from build123d import *

# Parameters (mm, degrees)
SKETCH1_W           = 70
SKETCH1_H           = 70
SKETCH1_R           = 3.1
BOSS_EXTRUDE1_DEPTH = 2
FILLET1_R           = 5
SKETCH2_R           = 10
BOSS_EXTRUDE2_DEPTH = 26
SKETCH5_R           = 6
CUT_EXTRUDE1_DEPTH  = 29
SKETCH6_R           = 7.5
CUT_EXTRUDE2_DEPTH  = 2


with BuildPart() as part:
    # Sketch1 → Boss-Extrude1 (new body)
    with BuildSketch(Plane(origin=(0, 0, 0), x_dir=(1, 0, 0), z_dir=(0, 1, 0))):
        Rectangle(SKETCH1_W, SKETCH1_H)
        with Locations((25, 25)):
            Circle(SKETCH1_R, mode=Mode.SUBTRACT)
        with Locations((-25, -25)):
            Circle(SKETCH1_R, mode=Mode.SUBTRACT)
        with Locations((-25, 25)):
            Circle(SKETCH1_R, mode=Mode.SUBTRACT)
        with Locations((25, -25)):
            Circle(SKETCH1_R, mode=Mode.SUBTRACT)
    extrude(amount=BOSS_EXTRUDE1_DEPTH)

    # Fillet1
    fillet1_edges = [part.edges().sort_by_distance(p)[0] for p in [
        (35, 1, 35),
        (-35, 1, 35),
        (-35, 1, -35),
        (35, 1, -35),
    ]]
    fillet(fillet1_edges, radius=FILLET1_R)

    # Sketch2 → Boss-Extrude2 (add)
    with BuildSketch(Plane.XZ):
        Circle(SKETCH2_R)
    extrude(amount=BOSS_EXTRUDE2_DEPTH)

    # Sketch5 → Cut-Extrude1 (cut, through all)
    with BuildSketch(Plane.XZ.offset(26)):
        Circle(SKETCH5_R)
    extrude(amount=-CUT_EXTRUDE1_DEPTH, mode=Mode.SUBTRACT)

    # Sketch6 → Cut-Extrude2 (cut)
    with BuildSketch(Plane(origin=(0, 2, 0), x_dir=(1, 0, 0), z_dir=(0, 1, 0))):
        Circle(SKETCH6_R)
    extrude(amount=-CUT_EXTRUDE2_DEPTH, mode=Mode.SUBTRACT)


solid = part.part
Design review of the part built by this model. Coordinates are the model's own, in mm. A direction names the side the tool comes from. Round coordinates to 2 decimals unless told otherwise and drop trailing zeros. Write each loop counter-clockwise with the first axis right and the second up, starting at its lowest first coordinate (ties: lowest second). Pieces come first, ordered by that corner, then holes.
Item 1: For faces 4 (the cylindrical face through (-7.493, 1.014, -0.33)), 5 (the cylindrical face through (-34, 1, -33)), 6 (the flat face through (7, 0, -8)), list the 3-axis set-ups (+Z, -Z, +X, -X, +Y, -Y) from which the entire face can be reached by the end or side of a thin tool; tool diameter is ignored.
Item 2: Draft analysis for pull direction Z (two halves, no side actions). For faces 1 (the flat face through (2, 0, -6)), 2 (the cylindrical face through (33, 1, 34)), 3 (the flat face through (35, 1, 0)), state which applies: released by +Z, released by -Z, zero draft, split by the parting line, or undercut.
Item 3: Consider section C-C on z = 0. Give the boundary of the cut face in (x, y).
Item 4: For pin 1 Ø10 at (x, z) = (25, -25) entering from -Y, flat-tipped, find the tip position at first contact; note if it passes through.
Item 5: Consider section A-A on z = -25. Give the boundary of the cut face in (x, y), and give its area (3 significant figures).
Item 6: Wall thickness on L1, parallel to Z at x = 25, y = 0.55; L2, parallel to Z at x = 0, y = 1.5: over which ranges is each line inside the solid? List them lowest first.
Item 7: Consider section D-D on x = -2. Give the boundary of the cut face in (y, z), and give its area (3 significant figures).
Item 8: Consider section B-B on x = -25. Give the boundary of the cut face in (y, z).
Check values:
1. face 4: +Y
1. face 5: -Z, -X, +Y, -Y
1. face 6: -Y
2. face 1: undercut
2. face 2: released by +Z
2. face 3: zero draft
3. outline: (-35, 0) - (-10, 0) - (-10, -26) - (-6, -26) - (-6, 0) - (-7.5, 0) - (-7.5, 2) - (-35, 2) - close; (6, -26) - (10, -26) - (10, 0) - (35, 0) - (35, 2) - (7.5, 2) - (7.5, 0) - (6, 0) - close
4. pin 1: stops at y = 0
5. outline: (-35, 0) - (-28.1, 0) - (-28.1, 2) - (-35, 2) - close; (-21.9, 0) - (21.9, 0) - (21.9, 2) - (-21.9, 2) - close; (28.1, 0) - (35, 0) - (35, 2) - (28.1, 2) - close
5. area: 115 mm2
6. L1: z = -35 to -28.1, -21.9 to 21.9, 28.1 to 35
6. L2: z = -35 to -7.5, 7.5 to 35
7. outline: (-26, -9.8) - (0, -9.8) - (0, -35) - (2, -35) - (2, -7.23) - (0, -7.23) - (0, -5.66) - (-26, -5.66) - close; (-26, 5.66) - (0, 5.66) - (0, 7.23) - (2, 7.23) - (2, 35) - (0, 35) - (0, 9.8) - (-26, 9.8) - close
7. area: 326 mm2
8. outline: (0, -35) - (2, -35) - (2, -28.1) - (0, -28.1) - close; (0, -21.9) - (2, -21.9) - (2, 21.9) - (0, 21.9) - close; (0, 28.1) - (2, 28.1) - (2, 35) - (0, 35) - close
